Drawing for the job (mm, zero at the part's lowest x, y, z). Round coordinates to 2 decimals unless told otherwise and drop trailing zeros. Order: outer loops, then holes, each group sorted by start corner. A loop starts at its lowest first (then second) coordinate and runs counter-clockwise, first axis right, second up. Notation, with made-up numbers: M 61,-37.75 L 120,-37.75 A16 cw 120,-14.75 Z; hole C 77,-11.75 d6. An arc over 180 degrees is marked long. Answer as CSV lines item,"result". Start each with the question number.
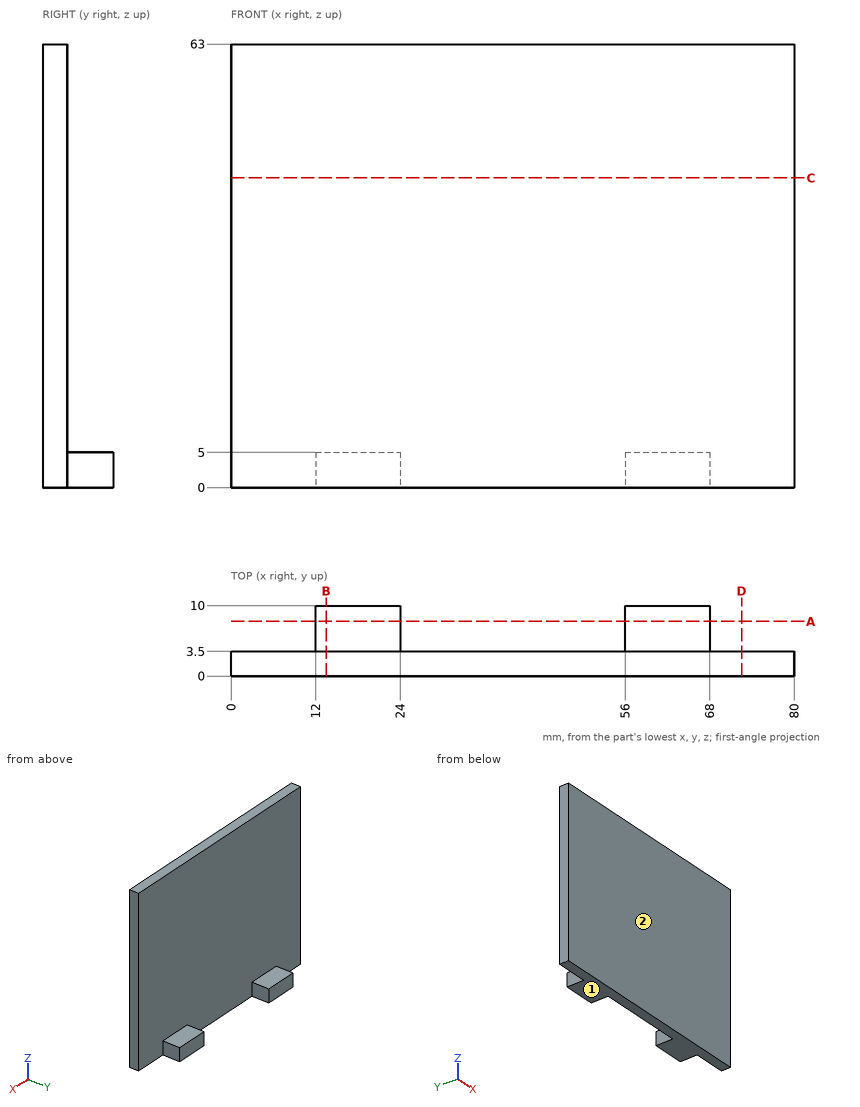
Q1. Mould opens along Y. For the marked faces 1 and 2 say: +Y half, -Y half, draft (parallel to the pull), parting line (faces both ways), or undercut.
Q2. Band-saw the part on B-B, the plane x = 13.5. Write the cut outline in (y, z), then the cut area to 3 significant figures.
Q3. Band-saw the part on A-A, the plane y = 7.75. Write the cut outline in (x, z).
Q4. Drop flat-ended pins along their axis: P1, Ø2, axis at y = 2, z = 24, coming from the -X side; P2, Ø3, axis at x = 65, z = 38, coming from the +Y side; P3, Ø3, axis at x = 19.5, y = 5.5, coming from the +Z side; P4, Ø1.5, axis at x = 36, y = 5, coming from the -Z side. Give the stop position or say it passes through.
Q5. Band-saw the part on D-D, the plane x = 72.5. Write the cut outline in (y, z), then the cut area to 4 significant figures.
Q6. Probe line 1 along Y through (x, z) = (66, 20); line 2 along Z through (x, y) = (15, 8.5). List the from-to ranges inside material, lowest first. Write a range as from..to.
Q7. Band-saw the part on C-C, the plane z = 44. Write the cut outline in (x, y).
Answer:
1,face 1,"draft"
1,face 2,"-Y half"
2,outline,"M 0,0 L 10,0 L 10,5 L 3.5,5 L 3.5,63 L 0,63 Z"
2,area,"253 mm^2"
3,outline,"M 12,0 L 24,0 L 24,5 L 12,5 Z; M 56,0 L 68,0 L 68,5 L 56,5 Z"
4,P1,"stops at x = 0"
4,P2,"stops at y = 3.5"
4,P3,"stops at z = 5"
4,P4,"passes through"
5,outline,"M 0,0 L 3.5,0 L 3.5,63 L 0,63 Z"
5,area,"220.5 mm^2"
6,line 1,"y = 0..3.5"
6,line 2,"z = 0..5"
7,outline,"M 0,0 L 80,0 L 80,3.5 L 0,3.5 Z"
